Can you work these out from the model? Positions are in its coordinate system, mm. A direction names the side the tool comes from. Round coordinates to 2 decimals unless told otherwise and drop trailing zeros. Order: outer loops, then holes, each group sorted by start corner. A loop starts at its lowest first (then second) coordinate and runs counter-clockwise, first axis right, second up. Notation, with made-up numbers: M 73,80.5 L 88,80.5 A26 cw 88,102.5 Z; hole C -30,44 d5. An arc over 180 degrees is marked long. One line per question, with ' | ' between items.
```python
from build123d import *

# Parameters (mm, degrees)
BOSS_EXTRUDE1_DEPTH = 1.25
SKETCH4_W           = 1
SKETCH4_H           = 1.325
BOSS_EXTRUDE4_DEPTH = 2
SKETCH5_W           = 1
SKETCH5_H           = 1.325
BOSS_EXTRUDE5_DEPTH = 2


with BuildPart() as part:
    # Sketch1 → Boss-Extrude1 (new body)
    with BuildSketch(Plane.XY):
        Polygon((1, 0), (9, 0), (9, -0.325), (10, -0.325), (10, -1), (17, -1), (17, 1), (10, 1), (0, 1), (-7, 1), (-7, -1), (0, -1), (0, -0.325), (1, -0.325), align=None)
    extrude(amount=BOSS_EXTRUDE1_DEPTH)

    # Sketch4 → Boss-Extrude4 (add)
    with BuildSketch(Plane(origin=(0, 0, 0), x_dir=(-1, 0, 0), z_dir=(0, 0, -1))):
        with Locations((-9.5, 0.3375)):
            Rectangle(SKETCH4_W, SKETCH4_H)
        with Locations((-0.5, 0.3375)):
            Rectangle(SKETCH4_W, SKETCH4_H)
    extrude(amount=BOSS_EXTRUDE4_DEPTH)

    # Sketch5 → Boss-Extrude5 (add)
    with BuildSketch(Plane.XY.offset(1.25)):
        with Locations((0.5, 0.3375)):
            Rectangle(SKETCH5_W, SKETCH5_H)
        with Locations((9.5, 0.3375)):
            Rectangle(SKETCH5_W, SKETCH5_H)
    extrude(amount=BOSS_EXTRUDE5_DEPTH)


solid = part.part
```
(1) Will these pins go through, and if not, where does the flat tip stop? pin 1 Ø1.1 at (y, z) = (0.5, 2) entering from +X; pin 2 Ø1.4 at (x, z) = (4, 0.5) entering from -Y; pin 3 Ø1.1 at (x, y) = (3.5, 0.5) entering from -Z.
Final values:
pin 1: x = 10 | pin 2: y = 0 | pin 3: z = 0
(2) If we section it at C-C on y = 0.25: Please give me the cut outline in (x, z), plus the area to 3 significant figures.
Final values:
outline: M -7,0 L 0,0 L 0,-2 L 1,-2 L 1,0 L 9,0 L 9,-2 L 10,-2 L 10,0 L 17,0 L 17,1.25 L 10,1.25 L 10,3.25 L 9,3.25 L 9,1.25 L 1,1.25 L 1,3.25 L 0,3.25 L 0,1.25 L -7,1.25 Z | area: 38.0 mm^2
(3) If we section it at D-D on x = 5.25: Please give me the cut outline in (y, z), plus the area to 3 significant figures.
Final values:
outline: M 0,0 L 1,0 L 1,1.25 L 0,1.25 Z | area: 1.25 mm^2
(4) On a 3-axis mill with a long thin cutter (end or side, diameter ignored), from which of +Z, -Z, +X, -X, +Y, -Y can I reach the whole of each face in a straight line? I mean faces 1 (the flat face through (4.9, 0.5, 0)), 2 (the flat face through (10, 0, 2)), 3 (the flat face through (4.9, 0.5, 1.25)), 4 (the flat face through (9.5, -0.325, 0.7)). Say none if no direction works.
Final values:
face 1: -Z, +Y, -Y | face 2: +Z, +X, +Y, -Y | face 3: +Z, +Y, -Y | face 4: +Z, -Z, -Y
(5) If we section it at A-A on z = 1.8: Please give me the cut outline in (x, y) (3 decimals), plus the area to 3 significant figures.
Final values:
outline: M 0,-0.325 L 1,-0.325 L 1,1 L 0,1 Z; M 9,-0.325 L 10,-0.325 L 10,1 L 9,1 Z | area: 2.65 mm^2
(6) Thinking about a two-plate mould opening in X: for faces 5 (the flat face through (0.5, -0.325, 0.6)), 6 (the flat face through (0, 0, -1)), 7 (the flat face through (-4, 0, 0)), which applies, released by +X, released by -X, zero draft, split by the parting line, or undercut?
Final values:
face 5: undercut | face 6: released by -X | face 7: zero draft
(7) Please list where these lines run through material, in increasing order: probe 1 along X at (y, z) = (-0.7, 0.3); probe 2 along X at (y, z) = (-0.1, -1.4); probe 3 along Y at (x, z) = (3.25, 0.8). Write a range as [from, to].
Final values:
probe 1: [-7, 0], [10, 17] | probe 2: [0, 1], [9, 10] | probe 3: [0, 1]
(8) If we section it at B-B on z = 0.6: Please give me the cut outline in (x, y) (3 decimals).
Final values:
outline: M -7,-1 L 0,-1 L 0,-0.325 L 1,-0.325 L 1,0 L 9,0 L 9,-0.325 L 10,-0.325 L 10,-1 L 17,-1 L 17,1 L -7,1 Z
